For this review, take the finished solid that the model builds, in its own axes (mm). A direction names the side the tool comes from. Coordinates: 2 decimals unless noted, no trailing zeros. Order: outer loops, then holes, each group sorted by start corner. A loop starts at its lowest first (then second) coordinate and runs counter-clockwise, first axis right, second up. Notation, with made-up numbers: (73.5, 17.5) -> (124.5, 17.5) arc R25 cw to (124.5, 55.5) -> close; hole circle Ø5 at (80, 29.5). An arc over 180 degrees is marked (long way). Answer as a JSON object with one key per item and string values. Group by question number.
1) Machinability: for faces 1 (the flat face through (-35, -10.553, -5)), 2 (the flat face through (124, 12.947, -4)), 3 (the flat face through (6, 3, -25)), 4 (the cylindrical face through (126.97, -46.08, 7.42)), which of the approach directions +Z, -Z, +X, -X, +Y, -Y give a long, thin tool a straight path to every point of the face, cutting with its end or side? Answer none if there is none.
2) Add section D-D, the plane y = -24.5. Write out the cut boundary in (x, z).
3) Add section B-B, the plane z = -4.5. Write out the cut boundary in (x, y), then the cut area to 3 significant figures.
4) Add section C-C, the plane x = 87. Write out the cut boundary in (y, z), then the cut area to 3 significant figures.
5) Draft analysis for pull direction X (two halves, no side actions). For faces 5 (the cylindrical face through (122.4, 20.1, 7.4)), 6 (the flat face through (95, -14, -32)), 7 (the flat face through (129.761, -12, -3)), 8 (the flat face through (-50.239, -16, -5)), state which applies: +X half, -X half, draft (parallel to the pull), parting line (faces both ways), or undercut.
6) For pin 1 (1 mm diameter, centred on y = -20, z = -13, fed in from -X); pin 2 (8 mm diameter, centred on x = -44, y = 10.5, fed in from +Z); pin 3 (2 mm diameter, centred on x = 25, y = 6.5, fed in from -Z), all flat-tipped, find the tip position at first contact; note any pin that passes through.
7) Wall thickness on L1, parallel to Z at x = -36, y = 9.5; L2, parallel to X at y = -26.5, z = -27.5; L3, parallel to Z at x = 87, y = 13: over which ranges is each line inside the solid? List them lowest first.
8) Add section A-A, the plane y = -14. Write out the cut boundary in (x, z).
from build123d import *

# Parameters (mm, degrees)
SKETCH1_W           = 165
SKETCH1_H           = 76
BOSS_EXTRUDE1_DEPTH = 1.5
CUT_EXTRUDE1_REACH  = 140.731
SKETCH2_R           = 1.5
SKETCH3_W           = 12
SKETCH3_H           = 40
BOSS_EXTRUDE2_DEPTH = 8
SKETCH4_W           = 50
SKETCH4_H           = 50
BOSS_EXTRUDE3_DEPTH = 32
SKETCH5_W           = 30
SKETCH5_H           = 10
BOSS_EXTRUDE4_DEPTH = 11
SKETCH6_R           = 6
BOSS_EXTRUDE5_DEPTH = 25
SKETCH7_R           = 3
BOSS_EXTRUDE6_DEPTH = 12


with BuildPart() as part:
    # Sketch1 → Boss-Extrude1 (new body)
    with BuildSketch(Plane.XY):
        with Locations((47.261306533, -11.052763819)):
            Rectangle(SKETCH1_W, SKETCH1_H)
    extrude(amount=BOSS_EXTRUDE1_DEPTH)

    # Sketch2 → Cut-Extrude1 (cut, up to next)
    with BuildSketch(Plane.XY.offset(1.5), mode=Mode.PRIVATE) as cut_extrude1_sk1:
        with Locations((124.761306533, 21.947236181)):
            Circle(SKETCH2_R)
    cut_extrude1_tool1 = extrude(cut_extrude1_sk1.sketch, amount=-CUT_EXTRUDE1_REACH, mode=Mode.PRIVATE) & part.part
    # Sketch2 → Cut-Extrude1 (cut, up to next)
    with BuildSketch(Plane.XY.offset(1.5), mode=Mode.PRIVATE) as cut_extrude1_sk2:
        with Locations((124.761306533, -44.052763819)):
            Circle(SKETCH2_R)
    cut_extrude1_tool2 = extrude(cut_extrude1_sk2.sketch, amount=-CUT_EXTRUDE1_REACH, mode=Mode.PRIVATE) & part.part
    # Sketch2 → Cut-Extrude1 (cut, up to next)
    with BuildSketch(Plane.XY.offset(1.5), mode=Mode.PRIVATE) as cut_extrude1_sk3:
        with Locations((-30.238693467, -44.052763819)):
            Circle(SKETCH2_R)
    cut_extrude1_tool3 = extrude(cut_extrude1_sk3.sketch, amount=-CUT_EXTRUDE1_REACH, mode=Mode.PRIVATE) & part.part
    # Sketch2 → Cut-Extrude1 (cut, up to next)
    with BuildSketch(Plane.XY.offset(1.5), mode=Mode.PRIVATE) as cut_extrude1_sk4:
        with Locations((-30.238693467, 21.947236181)):
            Circle(SKETCH2_R)
    cut_extrude1_tool4 = extrude(cut_extrude1_sk4.sketch, amount=-CUT_EXTRUDE1_REACH, mode=Mode.PRIVATE) & part.part
    add(cut_extrude1_tool1.solids().sort_by_distance((124.761307, 21.947236, 1.5))[0], mode=Mode.SUBTRACT)
    add(cut_extrude1_tool2.solids().sort_by_distance((124.761307, -44.052764, 1.5))[0], mode=Mode.SUBTRACT)
    add(cut_extrude1_tool3.solids().sort_by_distance((-30.238693, -44.052764, 1.5))[0], mode=Mode.SUBTRACT)
    add(cut_extrude1_tool4.solids().sort_by_distance((-30.238693, 21.947236, 1.5))[0], mode=Mode.SUBTRACT)

    # Sketch3 → Boss-Extrude2 (add)
    with BuildSketch(Plane(origin=(0, 0, 0), x_dir=(-1, 0, 0), z_dir=(0, 0, -1))):
        with Locations((-123.761306533, -7.052763819)):
            Rectangle(SKETCH3_W, SKETCH3_H)
    extrude(amount=BOSS_EXTRUDE2_DEPTH)

    # Sketch4 → Boss-Extrude3 (add)
    with BuildSketch(Plane(origin=(0, 0, 0), x_dir=(-1, 0, 0), z_dir=(0, 0, -1))):
        with Locations((-94.761306533, -14.052763819)):
            Rectangle(SKETCH4_W, SKETCH4_H)
    extrude(amount=BOSS_EXTRUDE3_DEPTH)

    # Sketch5 → Boss-Extrude4 (add)
    with BuildSketch(Plane(origin=(0, 0, 0), x_dir=(-1, 0, 0), z_dir=(0, 0, -1))):
        with Locations((35.238693467, 10.947236181)):
            Rectangle(SKETCH5_W, SKETCH5_H)
        with Locations((35.238693467, -15.552763819)):
            Rectangle(SKETCH5_W, SKETCH5_H)
    extrude(amount=BOSS_EXTRUDE4_DEPTH)

    # Sketch6 → Boss-Extrude5 (add)
    with BuildSketch(Plane(origin=(0, 0, 0), x_dir=(-1, 0, 0), z_dir=(0, 0, -1))):
        with Locations(Location((-5.761306533, 2.947236181, 0), (0, 0, 180))):
            Circle(SKETCH6_R)
    extrude(amount=BOSS_EXTRUDE5_DEPTH)

    # Sketch7 → Boss-Extrude6 (add)
    with BuildSketch(Plane.XY.offset(1.5)):
        with Locations((124.761306533, 21.947236181)):
            Circle(SKETCH7_R)
        with Locations(Location((124.761306533, -44.052763819, 0), (0, 0, 180))):
            Circle(SKETCH7_R)
        with Locations(Location((-30.238693467, 21.947236181, 0), (0, 0, 180))):
            Circle(SKETCH7_R)
        with Locations((-30.238693467, -44.052763819)):
            Circle(SKETCH7_R)
    extrude(amount=BOSS_EXTRUDE6_DEPTH)


solid = part.part
Output values:
{
 "1": {"face 1": "-Z, -X", "face 2": "-Z, +X, +Y", "face 3": "-Z, -X, +Y, -Y", "face 4": "+Z"},
 "2": {"outline": "(-35.24, 0) -> (69.76, 0) -> (69.76, -32) -> (119.76, -32) -> (119.76, -8) -> (129.76, -8) -> (129.76, 1.5) -> (-35.24, 1.5) -> close"},
 "3": {"outline": "(-50.24, -20.55) -> (-20.24, -20.55) -> (-20.24, -10.55) -> (-50.24, -10.55) -> close; (-50.24, 5.95) -> (-20.24, 5.95) -> (-20.24, 15.95) -> (-50.24, 15.95) -> close; circle Ø12 at (5.76, 2.95); (69.76, -39.05) -> (119.76, -39.05) -> (119.76, -27.05) -> (129.76, -27.05) -> (129.76, 12.95) -> (117.76, 12.95) -> (117.76, 10.95) -> (69.76, 10.95) -> close", "area": "3,620 mm²"},
 "4": {"outline": "(-49.05, 0) -> (-39.05, 0) -> (-39.05, -32) -> (10.95, -32) -> (10.95, 0) -> (26.95, 0) -> (26.95, 1.5) -> (-49.05, 1.5) -> close", "area": "1,710 mm²"},
 "5": {"face 5": "undercut", "face 6": "draft", "face 7": "+X half", "face 8": "-X half"},
 "6": {"pin 1": "stops at x = 69.76", "pin 2": "stops at z = 0", "pin 3": "stops at z = 0"},
 "7": {"L1": "z = -11 to 0", "L2": "x = 69.76 to 119.76", "L3": "z = 0 to 1.5"},
 "8": {"outline": "(-50.24, -11) -> (-20.24, -11) -> (-20.24, 0) -> (69.76, 0) -> (69.76, -32) -> (119.76, -32) -> (119.76, -8) -> (129.76, -8) -> (129.76, 1.5) -> (-35.24, 1.5) -> (-35.24, 0) -> (-50.24, 0) -> close"}
}
